from build123d import *

# Parameters (mm, degrees)
F0_W     = 11
F0_H     = 30
F1_DEPTH = 24
F3_DEPTH = 11
F4_R     = 2.5
F4_R_2   = 5
F5_DEPTH = 41.001
F6_R     = 13
F7_R     = 5
F8_R     = 2
F9_DEPTH = 11.3


with BuildPart() as f1:
    # F0 (on Right) → F1 (new body, symmetric)
    with BuildSketch(Plane.YZ):
        with BuildLine():
            Line((-56, 0), (-30, 0))
            ThreePointArc((-30, 0), (-29.4730143031, 5.5983415304), (-27.9105714739, 11))
            Line((-27.9105714739, 11), (-56, 11))
            Line((-56, 11), (-56, 0))
        make_face()
        with BuildLine():
            Line((-30, 0), (-19, 0))
            ThreePointArc((-19, 0), (-18.1017503893, 5.7729223833), (-15.4919333848, 11))
            Line((-15.4919333848, 11), (-27.9105714739, 11))
            ThreePointArc((-27.9105714739, 11), (-29.4730143031, 5.5983415304), (-30, 0))
        make_face()
        with BuildLine():
            ThreePointArc((15.4919333848, 11), (18.1017503893, 5.7729223833), (19, 0))
            Line((19, 0), (30, 0))
            ThreePointArc((30, 0), (29.4730143031, 5.5983415304), (27.9105714739, 11))
            Line((27.9105714739, 11), (15.4919333848, 11))
        make_face()
        with BuildLine():
            ThreePointArc((-15.4919333848, 11), (0, 19), (15.4919333848, 11))
            Line((15.4919333848, 11), (27.9105714739, 11))
            ThreePointArc((27.9105714739, 11), (0, 30), (-27.9105714739, 11))
            Line((-27.9105714739, 11), (-15.4919333848, 11))
        make_face()
        with BuildLine():
            ThreePointArc((27.9105714739, 11), (29.4730143031, 5.5983415304), (30, 0))
            Line((30, 0), (51, 0))
            Line((51, 0), (51, 11))
            Line((51, 11), (40, 11))
            Line((40, 11), (27.9105714739, 11))
        make_face()
        with Locations((45.5, 26)):
            Rectangle(F0_W, F0_H)
    extrude(amount=F1_DEPTH, both=True)

    # F2 (on face) → F3 (cut, through all)
    with BuildSketch(Plane(origin=(0, 51, 0), x_dir=(-1, 0, 0), z_dir=(0, 1, 0))):
        with BuildLine():
            ThreePointArc((-6.5, 25), (0, 18.5), (6.5, 25))
            ThreePointArc((6.5, 25), (0, 31.5), (-6.5, 25))
        make_face()
        with BuildLine():
            ThreePointArc((-6.5, 25), (0, 31.5), (6.5, 25))
            Line((6.5, 25), (6.5, 41))
            Line((6.5, 41), (-6.5, 41))
            Line((-6.5, 41), (-6.5, 25))
        make_face()
    extrude(amount=-F3_DEPTH, mode=Mode.SUBTRACT)

    # F4 (on Top) → F5 (cut, through all)
    with BuildSketch(Plane.XY):
        Circle(F4_R)
        with Locations((-11, -41.955285737)):
            Circle(F4_R_2)
        with Locations((11, -41.955285737)):
            Circle(F4_R_2)
    extrude(amount=F5_DEPTH, mode=Mode.SUBTRACT)

    # F6
    f6_edges = [f1.edges().sort_by_distance(p)[0] for p in [
        (24, -56, 5.5),
        (-24, -56, 5.5),
    ]]
    fillet(f6_edges, radius=F6_R)

    # F7
    f7_edges = [f1.edges().sort_by_distance(p)[0] for p in [
        (24, 45.5, 41),
        (-24, 45.5, 41),
    ]]
    fillet(f7_edges, radius=F7_R)

    # F8
    f8_edges = [f1.edges().sort_by_distance(p)[0] for p in [
        (0, -27.910571, 11),
        (0, 27.910571, 11),
    ]]
    fillet(f8_edges, radius=F8_R)

    # F9 (add): a face of the model
    f9_faces = [f1.faces().sort_by_distance(p)[0] for p in [
        (0, -41.9988312455, 11),
    ]]
    extrude(f9_faces, amount=F9_DEPTH)


solid = f1.part
The listing builds one solid part. Answer for the finished solid, in the listing's coordinates (mm). A direction names the side the tool comes from. Round coordinates to 2 decimals unless told otherwise and drop trailing zeros. Write each loop counter-clockwise with the first axis right and the second up, starting at its lowest first coordinate (ties: lowest second). Pieces come first, ordered by that corner, then holes. Notation, with made-up numbers: M 1,-0.5 L 28,-0.5 A37 cw 28,37.5 Z; hole C 27,-18.5 d2. An arc over 180 degrees is marked long. Write each question's results on one line, items separated by ' | '. Start each with the question number.
Item 1: A cutting plane is placed at D-D on x = 20.5. Write down the section's boundary in (y, z).
Item 2: A cutting plane is placed at C-C on z = 26.5. Write down the section's boundary in (x, y), and give its area (3 significant figures).
Item 3: A cutting plane is placed at B-B on z = 7. Write down the section's boundary in (x, y), and give its area (3 significant figures).
Item 4: For faces 1 (the face through (-6.5, 46, 33)), 2 (the face through (6, 40, 19)), 3 (the face through (23, 46, 39)), determine the directions among +Z, -Z, +X, -X, +Y, -Y from which every point of the face is accessible in a straight line to the end or side of a thin tool.
Item 5: A cutting plane is placed at A-A on x = -7.5. Write down the section's boundary in (y, z), and give its area (3 significant figures).
Item 6: Straight lines are drawn through the part: L1, parallel to Y at x = 0, z = 22; L2, parallel to Y at x = -19.5, z = 14; L3, parallel to Y at x = 8, z = 8. For each, find the intervals that lie inside material, in ascending order. Write a range as [from, to].
Item 7: Flat-ended cylindrical pins translate along their axes: pin 1 Ø21.5 at (x, y) = (-6.5, -40) entering from +Z; pin 2 Ø4 at (x, y) = (15.5, -2) entering from +Z; pin 3 Ø8 at (x, y) = (-11, -41.96) entering from +Z; pin 4 Ø4 at (x, z) = (11, 28) entering from -Y. Find the tip coordinate at first contact, or state that the pin passes through.
Check sheet entries:
1) outline: M -51.87,0 L -19,0 A19 cw 19,0 L 51,0 L 51,40.77 L 40,40.77 L 40,11 L 29.24,11 A2 cw 27.41,12.19 A30 ccw -27.41,12.19 A2 cw -29.24,11 L -29.24,22.3 L -51.87,22.3 Z
2) outline: M -24,-14.06 L 24,-14.06 L 24,14.06 L -24,14.06 Z; M -24,40 L -6.5,40 L -6.5,51 L -24,51 Z; M 6.5,40 L 24,40 L 24,51 L 6.5,51 Z; hole C 0,0 d5 | area: 1,720 mm²
3) outline: M -24,-43 A13 ccw -11,-56 L 11,-56 A13 ccw 24,-43 L 24,-17.66 L -24,-17.66 Z; M -24,17.66 L 24,17.66 L 24,51 L -24,51 Z; hole C -11,-41.96 d10; hole C 11,-41.96 d10 | area: 3,210 mm²
4) face 1: +Z, +Y | face 2: +Z, +X, -X | face 3: +Z, +X, +Y, -Y
5) outline: M -56,0 L -45.53,0 L -45.53,22.3 L -56,22.3 Z; M -38.38,0 L -19,0 A19 cw 19,0 L 51,0 L 51,41 L 40,41 L 40,11 L 29.24,11 A2 cw 27.41,12.19 A30 ccw -27.41,12.19 A2 cw -29.24,11 L -29.24,22.3 L -38.38,22.3 Z | area: 1,850 mm²
6) L1: [-56, -29.24], [-20.4, -2.5], [2.5, 20.4] | L2: [-52.84, -29.24], [-26.53, -12.85], [12.85, 26.53], [40, 51] | L3: [-56, -45.96], [-37.96, -17.23], [17.23, 51]
7) pin 1: z = 22.3 | pin 2: z = 30 | pin 3: through | pin 4: y = -14.97
